Part model, mm, in its own coordinate system. Round coordinates to 2 decimals unless told otherwise and drop trailing zeros. Loops run counter-clockwise (first coordinate to the right, second up) from the corner with the lowest first, then second, coordinate; pieces in that order, holes last.
(1) Probe probe 1 along Z at (x, y) = (22.5, 0.05); probe 2 along Y at (x, z) = (6.25, -0.15); probe 3 along Y at (x, z) = (15.25, -0.8). List the from-to ranges inside material, lowest first.
(2) Cut at A-A on x = 21.5. List the corners of the cut face in (y, z), then the cut area to 3 significant figures.
(3) Flat gauge pins, fed straight in: pin 1 (1.5 mm diameter, centred on x = 6, z = 0, fed in from -Y); pin 2 (1 mm diameter, centred on x = 8, z = -0.5, fed in from +Y); pin 3 (0.5 mm diameter, centred on x = 0.5, y = 1, fed in from -Z). Where does each tip first touch, or does it go through?
Solid Edge part; units mm, degrees
sketch "Sketch1" plane through (0, 0, 0) normal (0, -1, 0) x (1, 0, 0)
  line L0 (12, 0.95) -> (1.25, 0.95)
  line L1 (1.25, 1.63) -> (1.25, 0.95)
  spline S0 degree 3 poles (0, 0) (0, 0.7831) (0.4356, 1.448) (1.25, 1.63) knots 0 0 0 0 1 1 1 1
  line L2 (25.75, 0) -> (25.75, 0.95)
  line L3 (25.75, 0.95) -> (12, 0.95)
revolve "RevolvedProtrusion1" add sketch "Sketch1" angle 360 about axis through (0, 0, 0) along (1, 0, 0)
sketch "Sketch2" plane through (0, 0, 0) normal (1, 0, 0) x (0, 0, 1)
  line L0 (-0.375, 1.9976) -> (0.375, 1.9976)
  line L1 (0.375, 1.9976) -> (0.375, 0.6495)
  arc A0 (0.375, 0.6495) -> (0.375, -0.6495) centre (0, 0) cw
  line L2 (0.375, -0.6495) -> (0.375, -1.9976)
  line L3 (0.375, -1.9976) -> (-0.375, -1.9976)
  line L4 (-0.375, -1.9976) -> (-0.375, -0.6495)
  line L5 (-0.375, 0.6495) -> (-0.375, 1.9976)
  arc A1 (-0.375, -0.6495) -> (-0.375, 0.6495) centre (0, 0) cw
extrude "Cutout1" cut sketch "Sketch2" along normal blind 0.6
fillet "Round_1" radius 0.15 2 edges at (1.25, 0, -1.63) (25.75, 0, -0.95)
properties material "Galvanized steel"
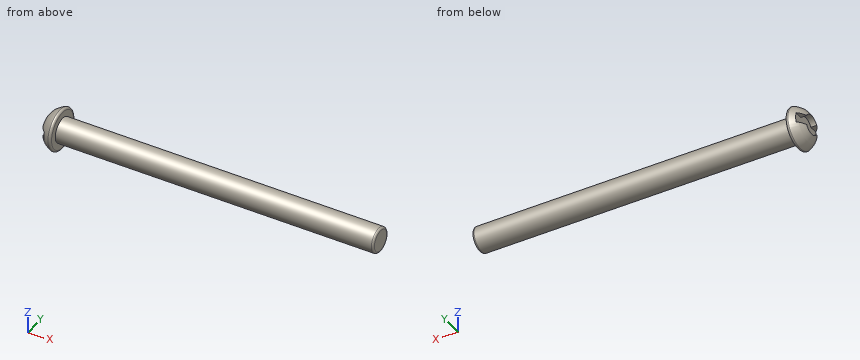
Final values:
1. probe 1: z = -0.95 to 0.95
1. probe 2: y = -0.94 to 0.94
1. probe 3: y = -0.51 to 0.51
2. outline: circle Ø1.9 at (0, 0)
2. area: 2.84 mm2
3. pin 1: stops at y = -0.95
3. pin 2: stops at y = 0.95
3. pin 3: stops at z = -1.12
